```python
from build123d import *

# Parameters (mm, degrees)
S_CYL1_R       = 19
BOSS_1_DEPTH   = 2.75
S_HOLE2_R      = 11.5
HOLE_2_DEPTH   = 2.95
S_CUT3_W       = 7.25
S_CUT3_H       = 40
POCKET_3_DEPTH = 2.95
S_CUT4_W       = 7.25
S_CUT4_H       = 40
POCKET_4_DEPTH = 2.95
S_CUT5_W       = 40
S_CUT5_H       = 9.45
POCKET_5_DEPTH = 2.95
S_CUT6_W       = 15
S_CUT6_H       = 11.9
POCKET_6_DEPTH = 1.65


with BuildPart() as part:
    # S_cyl1 → Boss_1 (new body)
    with BuildSketch(Plane.XY.offset(30.1)):
        Circle(S_CYL1_R)
    extrude(amount=BOSS_1_DEPTH)

    # S_hole2 → Hole_2 (cut)
    with BuildSketch(Plane.XY.offset(30)):
        with Locations(Location((0, 0, 0), (0, 0, 180))):
            Circle(S_HOLE2_R)
    extrude(amount=HOLE_2_DEPTH, mode=Mode.SUBTRACT)

    # S_cut3 → Pocket_3 (cut)
    with BuildSketch(Plane.XY.offset(30)):
        with Locations((16.375, 0)):
            Rectangle(S_CUT3_W, S_CUT3_H)
    extrude(amount=POCKET_3_DEPTH, mode=Mode.SUBTRACT)

    # S_cut4 → Pocket_4 (cut)
    with BuildSketch(Plane.XY.offset(30)):
        with Locations((-16.375, 0)):
            Rectangle(S_CUT4_W, S_CUT4_H)
    extrude(amount=POCKET_4_DEPTH, mode=Mode.SUBTRACT)

    # S_cut5 → Pocket_5 (cut)
    with BuildSketch(Plane.XY.offset(30)):
        with Locations((0, -15.275)):
            Rectangle(S_CUT5_W, S_CUT5_H)
    extrude(amount=POCKET_5_DEPTH, mode=Mode.SUBTRACT)

    # S_cut6 → Pocket_6 (cut)
    with BuildSketch(Plane.XY.offset(31.3)):
        with Locations((0, 14.05)):
            Rectangle(S_CUT6_W, S_CUT6_H)
    extrude(amount=POCKET_6_DEPTH, mode=Mode.SUBTRACT)


solid = part.part
```
Build history of the part. All positions in model axes, mm. A direction names the side the tool comes from. Give positions to 0.01 mm unless a question says otherwise; leave off trailing zeros. Loops run counter-clockwise (first coordinate to the right, second up) from the corner with the lowest first, then second, coordinate; pieces in that order, holes last. Notation, with made-up numbers: (-32, 46.5) -> (-26, 46.5) arc R26 ccw to (-26, 63.5) -> close; hole circle Ø3 at (14, 77.25). An arc over 180 degrees is marked (long way). One line per question, with ' | ' between items. Start each with the question number.
1) Cut at C-C (x = -10). Give the cut face in (y, z), plus the area to 3 significant figures.
2) Probe L1, parallel to X at y = 0, z = 31.2; L2, parallel to Z at x = -3, y = 16. List the from-to ranges inside material, lowest first.
3) Two-plate mould, pull along X, no slides. Class faces 3 (the cylindrical face through (0, 19, 31)), 4 (the flat face through (0, 14, 31.3)), 5 (the cylindrical face through (-7.849, -8.405, 31.456)), 6 (the flat face through (-9, -10.55, 31)): released by +X, released by -X, zero draft, split by the parting line, or undercut.
4) Cut at A-A (z = 32.15). Give the cut face in (x, y), plus the area to 3 significant figures.
5) Pin check, flat tip, straight feed: pin 1 (11.5 mm diameter, centred on x = 1, y = 12.5, fed in from +Z). Stop position of the tip, or through.
6) 3-axis set-ups, long thin cutter, end or side, ignore diameter. For faces 1 (the flat face through (7.5, 13, 32)), 2 (the flat face through (9, -10.55, 31)): which of +Z, -Z, +X, -X, +Y, -Y reach the whole face in a straight line?
7) Cut at D-D (x = 0). Give the cut face in (y, z), plus the area to 3 significant figures.
8) Cut at B-B (y = 0). Give the cut face in (x, z).
Return value:
1) outline: (-10.55, 30.1) -> (-5.68, 30.1) -> (-5.68, 32.85) -> (-10.55, 32.85) -> close; (5.68, 30.1) -> (16.16, 30.1) -> (16.16, 32.85) -> (5.68, 32.85) -> close | area: 42.2 mm^2
2) L1: -12.75 to -11.5, 11.5 to 12.75 | L2: 30.1 to 31.3
3) face 3: split by the parting line | face 4: undercut | face 5: undercut | face 6: zero draft
4) outline: (-12.75, -10.55) -> (-4.58, -10.55) arc R11.5 cw to (-7.5, 8.72) -> (-7.5, 17.46) arc R19 ccw to (-12.75, 14.09) -> close; (4.58, -10.55) -> (12.75, -10.55) -> (12.75, 14.09) arc R19 ccw to (7.5, 17.46) -> (7.5, 8.72) arc R11.5 cw to start | area: 186 mm^2
5) pin 1: z = 31.3
6) face 1: +Z, +Y | face 2: +Z, -Z, +X, -X, -Y
7) outline: (11.5, 30.1) -> (19, 30.1) -> (19, 31.3) -> (11.5, 31.3) -> close | area: 9.00 mm^2
8) outline: (-12.75, 30.1) -> (-11.5, 30.1) -> (-11.5, 32.85) -> (-12.75, 32.85) -> close; (11.5, 30.1) -> (12.75, 30.1) -> (12.75, 32.85) -> (11.5, 32.85) -> close
